Drawing for the job (mm, zero at the part's lowest x, y, z). A direction names the side the tool comes from. Coordinates: 2 decimals unless noted, no trailing zeros. Write each loop counter-clockwise with the first axis right and the second up, starting at its lowest first coordinate (ties: lowest second). Pieces come first, ordered by that corner, then holes. Notation, with made-up numbers: (18, 88) -> (70, 88) arc R13 ccw to (70, 95) -> close; hole circle Ø3 at (-29.75, 16.25). An arc over 180 degrees is marked (long way). Answer as CSV lines item,"result".
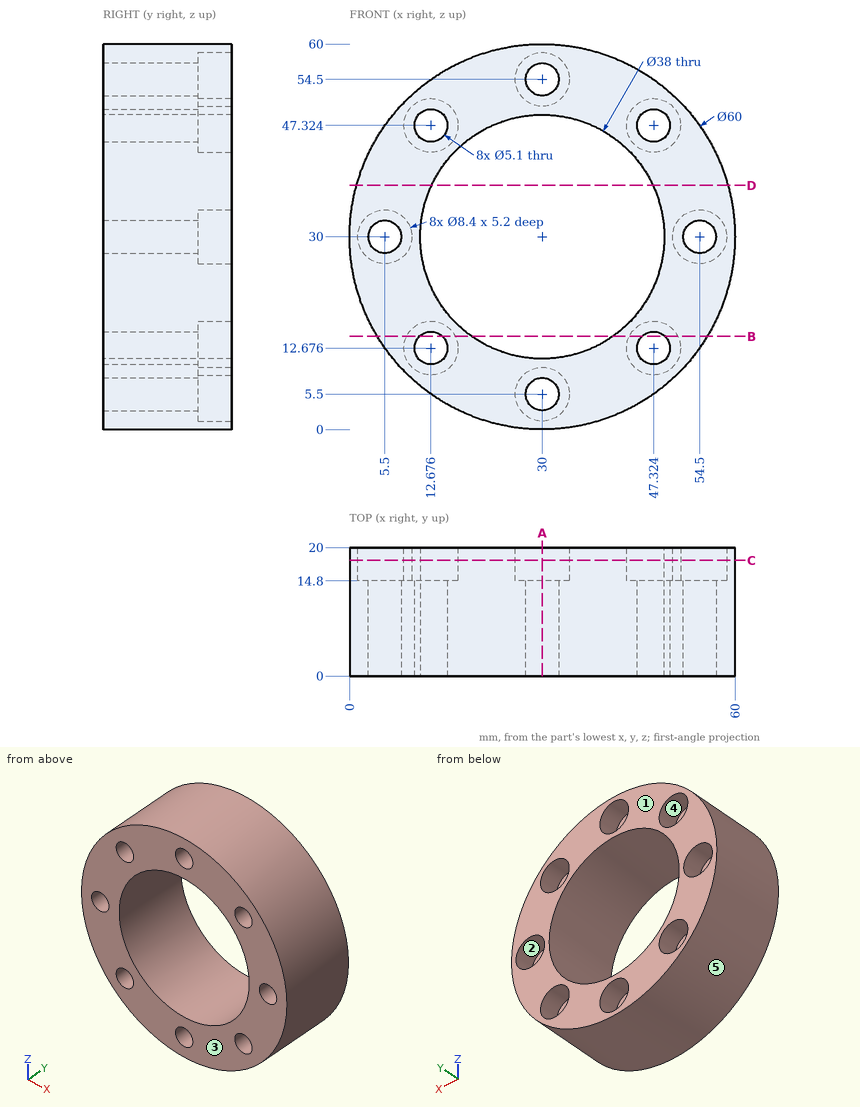
Item 1: Wall check: line 1 (X direction, y = 16.05, z = 30); line 2 (Z direction, x = 30, y = 8). Give the ranges that are in metal, low to high. Write a range as from..to.
Answer below:
line 1,"x = 0..1.3, 9.7..11, 49..50.3, 58.7..60"
line 2,"z = 0..2.95, 8.05..11, 49..51.95, 57.05..60"
Item 2: Saw through at C-C on y = 18. State how many separate pieces and enclosed holes the cut face has, and give its area (3 significant figures).
Answer below:
separate pieces,"1"
enclosed holes,"9"
area,"1,250 mm2"
Item 3: Two-plate mould, pull along Z, no slides. Class the marked faces 3, 4 and 5: pulls with the +Z half, pulls with the -Z half, needs draft (parallel to the pull), parting line crosses it, or undercut.
Answer below:
face 3,"needs draft"
face 4,"undercut"
face 5,"parting line crosses it"
Item 4: Saw through at B-B on z = 14.5. Give the cut face in (x, y), and give its area (3 significant figures).
Answer below:
outline,"(4.31, 0) -> (10.89, 0) -> (10.89, 14.8) -> (8.89, 14.8) -> (8.89, 20) -> (4.31, 20) -> close; (14.46, 0) -> (19.01, 0) -> (19.01, 20) -> (16.46, 20) -> (16.46, 14.8) -> (14.46, 14.8) -> close; (40.99, 0) -> (45.54, 0) -> (45.54, 14.8) -> (43.54, 14.8) -> (43.54, 20) -> (40.99, 20) -> close; (49.11, 0) -> (55.69, 0) -> (55.69, 20) -> (51.11, 20) -> (51.11, 14.8) -> (49.11, 14.8) -> close"
area,"404 mm2"
Item 5: Flat gauge pins, fed straight in: pin 1 (2 mm diameter, centred on x = 21.5, y = 11, fed in from -Z); pin 2 (5 mm diameter, centred on y = 12.5, z = 34.5, fed in from +X); pin 3 (6 mm diameter, centred on x = 30, z = 5.5, fed in from -Y); pin 4 (5 mm diameter, centred on y = 7.5, z = 33, fed in from +X). Where does each tip first touch, or does it go through?
Answer below:
pin 1,"stops at z = 0.95"
pin 2,"stops at x = 59.93"
pin 3,"stops at y = 0"
pin 4,"stops at x = 60"
Item 6: Saw through at D-D on z = 38. Give the cut face in (x, y).
Answer below:
outline,"(1.09, 0) -> (12.77, 0) -> (12.77, 20) -> (1.09, 20) -> close; (47.23, 0) -> (58.91, 0) -> (58.91, 20) -> (47.23, 20) -> close"
Item 7: Saw through at A-A on x = 30. Give the cut face in (y, z).
Answer below:
outline,"(0, 0) -> (20, 0) -> (20, 1.3) -> (14.8, 1.3) -> (14.8, 2.95) -> (0, 2.95) -> close; (0, 8.05) -> (14.8, 8.05) -> (14.8, 9.7) -> (20, 9.7) -> (20, 11) -> (0, 11) -> close; (0, 49) -> (20, 49) -> (20, 50.3) -> (14.8, 50.3) -> (14.8, 51.95) -> (0, 51.95) -> close; (0, 57.05) -> (14.8, 57.05) -> (14.8, 58.7) -> (20, 58.7) -> (20, 60) -> (0, 60) -> close"
Item 8: 3-axis set-ups, long thin cutter, end or side, ignore diameter. For the marked faces 1 and 2: which of +Z, -Z, +X, -X, +Y, -Y reach the whole face in a straight line?
Answer below:
face 1,"+Z, -Z, +X, -X, +Y"
face 2,"+Y"
